Model file for the job. Use its own axes, mm. A direction names the side the tool comes from. Coordinates: 2 decimals unless noted, no trailing zeros. Loops run counter-clockwise (first coordinate to the right, second up) from the corner with the lowest first, then second, coordinate; pieces in that order, holes last. Notation, with made-up numbers: (88.25, 34.5) -> (125.25, 34.5) arc R25 ccw to (125.25, 52.5) -> close; hole circle Ø5 at (24, 7). An arc over 180 degrees is marked (long way). Use one line per item in the form item = value.
```python
from build123d import *

# Parameters (mm, degrees)
F0_W     = 860
F0_H     = 80
F1_DEPTH = 300
F2_R     = 7.5
F3_DEPTH = 100
F5_DEPTH = 225
F6_R     = 10


with BuildPart() as f1:
    # F0 (on Top) → F1 (new body, symmetric)
    with BuildSketch(Plane.XY):
        with Locations((84.33931, -58.683639)):
            Rectangle(F0_W, F0_H)
    extrude(amount=F1_DEPTH, both=True)

    # F2 (on face) → F3 (join)
    with BuildSketch(Plane(origin=(0, 0, -300), x_dir=(1, 0, 0), z_dir=(0, 0, -1))):
        with Locations((494.33931, 58.683639)):
            Circle(F2_R)
        with Locations((-325.66069, 58.683639)):
            Circle(F2_R)
    extrude(amount=F3_DEPTH)

    # F4 (on Top) → F5 (cut, symmetric)
    with BuildSketch(Plane.XY):
        with BuildLine():
            Line((-265.66069, -18.683639), (-305.66069, -18.683639))
            Line((-305.66069, -18.683639), (-302.124776, -22.897577))
            ThreePointArc((-302.124776, -22.897577), (-300.407645, -24.215178), (-298.294554, -24.683639))
            Line((-298.294554, -24.683639), (-273.026826, -24.683639))
            ThreePointArc((-273.026826, -24.683639), (-270.913735, -24.215178), (-269.196604, -22.897577))
            Line((-269.196604, -22.897577), (-265.66069, -18.683639))
        make_face()
        with BuildLine():
            Line((-185.66069, -18.683639), (-225.66069, -18.683639))
            Line((-225.66069, -18.683639), (-222.124776, -22.897577))
            ThreePointArc((-222.124776, -22.897577), (-220.407645, -24.215178), (-218.294554, -24.683639))
            Line((-218.294554, -24.683639), (-193.026826, -24.683639))
            ThreePointArc((-193.026826, -24.683639), (-190.913735, -24.215178), (-189.196604, -22.897577))
            Line((-189.196604, -22.897577), (-185.66069, -18.683639))
        make_face()
        with BuildLine():
            Line((-105.66069, -18.683639), (-145.66069, -18.683639))
            Line((-145.66069, -18.683639), (-142.124776, -22.897577))
            ThreePointArc((-142.124776, -22.897577), (-140.407645, -24.215178), (-138.294554, -24.683639))
            Line((-138.294554, -24.683639), (-113.026826, -24.683639))
            ThreePointArc((-113.026826, -24.683639), (-110.913735, -24.215178), (-109.196604, -22.897577))
            Line((-109.196604, -22.897577), (-105.66069, -18.683639))
        make_face()
        with BuildLine():
            Line((-25.66069, -18.683639), (-65.66069, -18.683639))
            Line((-65.66069, -18.683639), (-62.124776, -22.897577))
            ThreePointArc((-62.124776, -22.897577), (-60.407645, -24.215178), (-58.294554, -24.683639))
            Line((-58.294554, -24.683639), (-33.026826, -24.683639))
            ThreePointArc((-33.026826, -24.683639), (-30.913735, -24.215178), (-29.196604, -22.897577))
            Line((-29.196604, -22.897577), (-25.66069, -18.683639))
        make_face()
        with BuildLine():
            Line((54.33931, -18.683639), (14.33931, -18.683639))
            Line((14.33931, -18.683639), (17.875224, -22.897577))
            ThreePointArc((17.875224, -22.897577), (19.592355, -24.215178), (21.705446, -24.683639))
            Line((21.705446, -24.683639), (46.973174, -24.683639))
            ThreePointArc((46.973174, -24.683639), (49.086265, -24.215178), (50.803396, -22.897577))
            Line((50.803396, -22.897577), (54.33931, -18.683639))
        make_face()
        with BuildLine():
            Line((134.33931, -18.683639), (94.33931, -18.683639))
            Line((94.33931, -18.683639), (97.875224, -22.897577))
            ThreePointArc((97.875224, -22.897577), (99.592355, -24.215178), (101.705446, -24.683639))
            Line((101.705446, -24.683639), (126.973174, -24.683639))
            ThreePointArc((126.973174, -24.683639), (129.086265, -24.215178), (130.803396, -22.897577))
            Line((130.803396, -22.897577), (134.33931, -18.683639))
        make_face()
        with BuildLine():
            Line((214.33931, -18.683639), (174.33931, -18.683639))
            Line((174.33931, -18.683639), (177.875224, -22.897577))
            ThreePointArc((177.875224, -22.897577), (179.592355, -24.215178), (181.705446, -24.683639))
            Line((181.705446, -24.683639), (206.973174, -24.683639))
            ThreePointArc((206.973174, -24.683639), (209.086265, -24.215178), (210.803396, -22.897577))
            Line((210.803396, -22.897577), (214.33931, -18.683639))
        make_face()
        with BuildLine():
            Line((294.33931, -18.683639), (254.33931, -18.683639))
            Line((254.33931, -18.683639), (257.875224, -22.897577))
            ThreePointArc((257.875224, -22.897577), (259.592355, -24.215178), (261.705446, -24.683639))
            Line((261.705446, -24.683639), (286.973174, -24.683639))
            ThreePointArc((286.973174, -24.683639), (289.086265, -24.215178), (290.803396, -22.897577))
            Line((290.803396, -22.897577), (294.33931, -18.683639))
        make_face()
        with BuildLine():
            Line((374.33931, -18.683639), (334.33931, -18.683639))
            Line((334.33931, -18.683639), (337.875224, -22.897577))
            ThreePointArc((337.875224, -22.897577), (339.592355, -24.215178), (341.705446, -24.683639))
            Line((341.705446, -24.683639), (366.973174, -24.683639))
            ThreePointArc((366.973174, -24.683639), (369.086265, -24.215178), (370.803396, -22.897577))
            Line((370.803396, -22.897577), (374.33931, -18.683639))
        make_face()
        with BuildLine():
            Line((454.33931, -18.683639), (414.33931, -18.683639))
            Line((414.33931, -18.683639), (417.875224, -22.897577))
            ThreePointArc((417.875224, -22.897577), (419.592355, -24.215178), (421.705446, -24.683639))
            Line((421.705446, -24.683639), (446.973174, -24.683639))
            ThreePointArc((446.973174, -24.683639), (449.086265, -24.215178), (450.803396, -22.897577))
            Line((450.803396, -22.897577), (454.33931, -18.683639))
        make_face()
        with BuildLine():
            ThreePointArc((-298.294554, -92.683639), (-300.407645, -93.1521), (-302.124776, -94.469701))
            Line((-302.124776, -94.469701), (-305.66069, -98.683639))
            Line((-305.66069, -98.683639), (-265.66069, -98.683639))
            Line((-265.66069, -98.683639), (-269.196604, -94.469701))
            ThreePointArc((-269.196604, -94.469701), (-270.913735, -93.1521), (-273.026826, -92.683639))
            Line((-273.026826, -92.683639), (-298.294554, -92.683639))
        make_face()
        with BuildLine():
            Line((-222.124776, -94.469701), (-225.66069, -98.683639))
            Line((-225.66069, -98.683639), (-185.66069, -98.683639))
            Line((-185.66069, -98.683639), (-189.196604, -94.469701))
            ThreePointArc((-189.196604, -94.469701), (-190.913735, -93.1521), (-193.026826, -92.683639))
            Line((-193.026826, -92.683639), (-218.294554, -92.683639))
            ThreePointArc((-218.294554, -92.683639), (-220.407645, -93.1521), (-222.124776, -94.469701))
        make_face()
        with BuildLine():
            ThreePointArc((290.803396, -94.469701), (289.086265, -93.1521), (286.973174, -92.683639))
            Line((286.973174, -92.683639), (261.705446, -92.683639))
            ThreePointArc((261.705446, -92.683639), (259.592355, -93.1521), (257.875224, -94.469701))
            Line((257.875224, -94.469701), (254.33931, -98.683639))
            Line((254.33931, -98.683639), (294.33931, -98.683639))
            Line((294.33931, -98.683639), (290.803396, -94.469701))
        make_face()
        with BuildLine():
            Line((-62.124776, -94.469701), (-65.66069, -98.683639))
            Line((-65.66069, -98.683639), (-25.66069, -98.683639))
            Line((-25.66069, -98.683639), (-29.196604, -94.469701))
            ThreePointArc((-29.196604, -94.469701), (-30.913735, -93.1521), (-33.026826, -92.683639))
            Line((-33.026826, -92.683639), (-58.294554, -92.683639))
            ThreePointArc((-58.294554, -92.683639), (-60.407645, -93.1521), (-62.124776, -94.469701))
        make_face()
        with BuildLine():
            Line((-105.66069, -98.683639), (-109.196604, -94.469701))
            ThreePointArc((-109.196604, -94.469701), (-110.913735, -93.1521), (-113.026826, -92.683639))
            Line((-113.026826, -92.683639), (-138.294554, -92.683639))
            ThreePointArc((-138.294554, -92.683639), (-140.407645, -93.1521), (-142.124776, -94.469701))
            Line((-142.124776, -94.469701), (-145.66069, -98.683639))
            Line((-145.66069, -98.683639), (-105.66069, -98.683639))
        make_face()
        with BuildLine():
            Line((417.875224, -94.469701), (414.33931, -98.683639))
            Line((414.33931, -98.683639), (454.33931, -98.683639))
            Line((454.33931, -98.683639), (450.803396, -94.469701))
            ThreePointArc((450.803396, -94.469701), (449.086265, -93.1521), (446.973174, -92.683639))
            Line((446.973174, -92.683639), (421.705446, -92.683639))
            ThreePointArc((421.705446, -92.683639), (419.592355, -93.1521), (417.875224, -94.469701))
        make_face()
        with BuildLine():
            Line((17.875224, -94.469701), (14.33931, -98.683639))
            Line((14.33931, -98.683639), (54.33931, -98.683639))
            Line((54.33931, -98.683639), (50.803396, -94.469701))
            ThreePointArc((50.803396, -94.469701), (49.086265, -93.1521), (46.973174, -92.683639))
            Line((46.973174, -92.683639), (21.705446, -92.683639))
            ThreePointArc((21.705446, -92.683639), (19.592355, -93.1521), (17.875224, -94.469701))
        make_face()
        with BuildLine():
            Line((134.33931, -98.683639), (130.803396, -94.469701))
            ThreePointArc((130.803396, -94.469701), (129.086265, -93.1521), (126.973174, -92.683639))
            Line((126.973174, -92.683639), (101.705446, -92.683639))
            ThreePointArc((101.705446, -92.683639), (99.592355, -93.1521), (97.875224, -94.469701))
            Line((97.875224, -94.469701), (94.33931, -98.683639))
            Line((94.33931, -98.683639), (134.33931, -98.683639))
        make_face()
        with BuildLine():
            ThreePointArc((370.803396, -94.469701), (369.086265, -93.1521), (366.973174, -92.683639))
            Line((366.973174, -92.683639), (341.705446, -92.683639))
            ThreePointArc((341.705446, -92.683639), (339.592355, -93.1521), (337.875224, -94.469701))
            Line((337.875224, -94.469701), (334.33931, -98.683639))
            Line((334.33931, -98.683639), (374.33931, -98.683639))
            Line((374.33931, -98.683639), (370.803396, -94.469701))
        make_face()
        with BuildLine():
            Line((177.875224, -94.469701), (174.33931, -98.683639))
            Line((174.33931, -98.683639), (214.33931, -98.683639))
            Line((214.33931, -98.683639), (210.803396, -94.469701))
            ThreePointArc((210.803396, -94.469701), (209.086265, -93.1521), (206.973174, -92.683639))
            Line((206.973174, -92.683639), (181.705446, -92.683639))
            ThreePointArc((181.705446, -92.683639), (179.592355, -93.1521), (177.875224, -94.469701))
        make_face()
    extrude(amount=F5_DEPTH, both=True, mode=Mode.SUBTRACT)

    # F6
    f6_edges = [f1.edges().sort_by_distance(p)[0] for p in [
        (-345.66069, -98.683639, 0),
        (-345.66069, -18.683639, 0),
        (514.33931, -98.683639, 0),
        (514.33931, -18.683639, 0),
        (84.33931, -98.683639, 300),
        (84.33931, -18.683639, 300),
        (514.33931, -58.683639, 300),
        (-345.66069, -58.683639, 300),
    ]]
    fillet(f6_edges, radius=F6_R)


solid = f1.part
```
Q1. Band-saw the part on A-A, the plane x = -284. Write the cut outline in (y, z).
Result:
outline = (-98.68, -300) -> (-18.68, -300) -> (-18.68, -225) -> (-24.68, -225) -> (-24.68, 225) -> (-18.68, 225) -> (-18.68, 290) arc R10 ccw to (-28.68, 300) -> (-88.68, 300) arc R10 ccw to (-98.68, 290) -> (-98.68, 225) -> (-92.68, 225) -> (-92.68, -225) -> (-98.68, -225) -> close
Q2. Band-saw the part on C-C, the plane x = 156.5. Write the cut outline in (y, z), and give its area (3 significant figures).
Result:
outline = (-98.68, -300) -> (-18.68, -300) -> (-18.68, 290) arc R10 ccw to (-28.68, 300) -> (-88.68, 300) arc R10 ccw to (-98.68, 290) -> close
area = 48,000 mm2
Q3. Pin check, flat tips, straight feed: pin 1 Ø1.8 at (x, y) = (123, -22) entering from +Z; pin 2 Ø20 at (x, z) = (350.5, -32.5) entering from -Y; pin 3 Ø7.5 at (x, z) = (277, -33) entering from -Y. Stop position of each tip, or through.
Result:
pin_1 = 298.16
pin_2 = -92.83
pin_3 = -92.68
Q4. Which spindle directions (+Z, -Z, +X, -X, +Y, -Y) get a long thin tool onto all of the face, cutting with end or side? Do faces 1 (the face through (514.339, -59, -1)), 2 (the face through (114, -24.684, -3)), 3 (the face through (-205, -92.684, -3)). Say none if no direction does.
Result:
face_1 = +Z, -Z, +X, +Y, -Y
face_2 = +Y
face_3 = -Y
Q5. Mould opens along Z. For faces 4 (the face through (78, -58, 300)), 5 (the face through (-345.661, -59, -1)), 6 (the face through (34, -24.684, -3)), 7 (the face through (-45, -92.684, -3)) say: released by +Z, released by -Z, zero draft, split by the parting line, or undercut.
Result:
face_4 = released by +Z
face_5 = zero draft
face_6 = undercut
face_7 = undercut
Q6. Band-saw the part on B-B, the plane z = -352. Write the cut outline in (x, y).
Result:
outline = circle Ø15 at (-325.66, -58.68); circle Ø15 at (494.34, -58.68)
Q7. Wall check: line 1 along Y through (x, z) = (266.5, 41); line 2 along Z through (x, y) = (-101.5, -27); line 3 along Z through (x, y) = (-41, -90.5). Give the ranges that are in metal, low to high.
Result:
line_1 = -92.68 to -24.68
line_2 = -300 to 299.86
line_3 = -300 to 299.83
